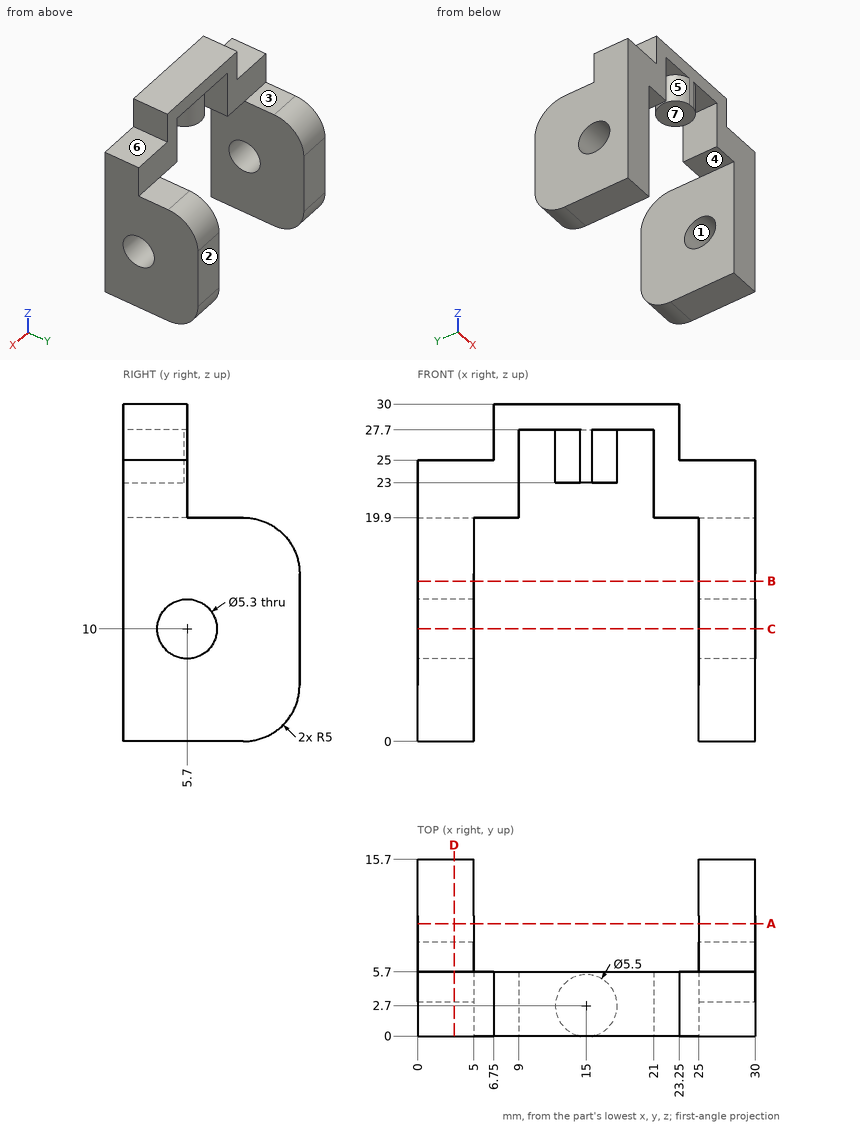
Input: dimensioned drawing with shaded views. Units: mm. Origin: part minimum x, y, z. A direction names the side the tool comes from. Round coordinates to 2 decimals unless told otherwise and drop trailing zeros. Order: outer loops, then holes, each group sorted by start corner. A loop starts at its lowest first (then second) coordinate and runs counter-clockwise, first axis right, second up. Notation, with made-up numbers: (38, -32) -> (54, -32) arc R4 ccw to (54, -27) -> close; hole circle Ø10 at (38.25, -3). An arc over 180 degrees is marked (long way). Put each result on its own line as item: value. Start each with the question number.
Q1. First-contact query: pin 1 (2.5 mm diameter, centred on x = 28, y = 9, fed in from +Z); pin 2 (8 mm diameter, centred on x = 19, z = 10, fed in from +Y); pin 3 (3 mm diameter, centred on x = 16, y = 2, fed in from -Z); pin 4 (5.5 mm diameter, centred on x = 3, y = 7, fed in from +Z). Flat tips, straight axial feed; report the tip coordinate or a pass-through.
Q2. Line query: probe 1 along X at (y, z) = (5.5, 21.25); probe 2 along X at (y, z) = (5, 5); probe 3 along Y at (x, z) = (8, 26.5). Output: solid intervals per line, ascending.
Q3. Section B-B on z = 14.25. Return the cut outline in (x, y).
Q4. Pull-direction query (Z, two-part tool) for the marked faces 1, 2, 3 and 4; classes: +Z half, -Z half, draft (parallel to the pull), parting line (faces both ways), or undercut.
Q5. Section C-C on z = 10. Return the cut outline in (x, y).
Q6. Section A-A on y = 10. Return the cut outline in (x, z).
Q7. Reachability of the marked faces 5, 6 and 7 from +Z, -Z, +X, -X, +Y, -Y: full face, straight path, thin tool, end or side. Return the list, or none.
Q8. Section D-D on x = 3.25. Return the cut outline in (y, z).
Ans:
1. pin 1: stops at z = 19.9
1. pin 2: passes through
1. pin 3: stops at z = 23
1. pin 4: stops at z = 25
2. probe 1: x = 0 to 9, 21 to 30
2. probe 2: x = 0 to 5, 25 to 30
2. probe 3: y = 0 to 5.7
3. outline: (0, 0) -> (5, 0) -> (5, 15.7) -> (0, 15.7) -> close; (25, 0) -> (30, 0) -> (30, 15.7) -> (25, 15.7) -> close
4. face 1: undercut
4. face 2: draft
4. face 3: +Z half
4. face 4: -Z half
5. outline: (0, 0) -> (5, 0) -> (5, 3.05) -> (0, 3.05) -> close; (0, 8.35) -> (5, 8.35) -> (5, 15.7) -> (0, 15.7) -> close; (25, 0) -> (30, 0) -> (30, 3.05) -> (25, 3.05) -> close; (25, 8.35) -> (30, 8.35) -> (30, 15.7) -> (25, 15.7) -> close
6. outline: (0, 0) -> (5, 0) -> (5, 19.9) -> (0, 19.9) -> close; (25, 0) -> (30, 0) -> (30, 19.9) -> (25, 19.9) -> close
7. face 5: -Z
7. face 6: +Z, +X, +Y, -Y
7. face 7: -Z, +Y, -Y
8. outline: (0, 0) -> (10.7, 0) arc R5 ccw to (15.7, 5) -> (15.7, 14.9) arc R5 ccw to (10.7, 19.9) -> (5.7, 19.9) -> (5.7, 25) -> (0, 25) -> close; hole circle Ø5.3 at (5.7, 10)
